Drawing for the job (mm, zero at the part's lowest x, y, z). Coordinates: 2 decimals unless noted, no trailing zeros. Write each loop counter-clockwise with the first axis right and the second up, starting at its lowest first coordinate (ties: lowest second). Pieces come first, ordered by that corner, then holes. Notation, with made-up numbers: (54, 44.5) -> (61, 44.5) arc R27 ccw to (61, 60.5) -> close; hole circle Ø9 at (69, 75). An arc over 180 degrees is marked (long way). Answer as CSV lines item,"result".
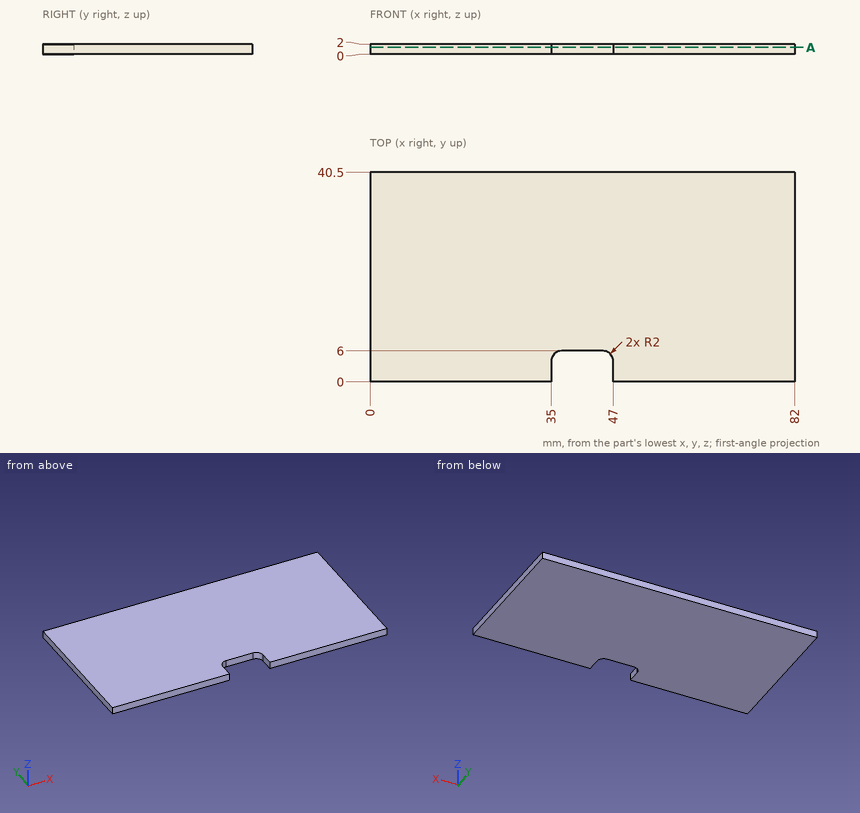
Item 1: Saw through at A-A on z = 1.35. Give the cut face in (x, y), and give its area (3 significant figures).
Answer below:
outline,"(0, 0) -> (35, 0) -> (35, 4) arc R2 cw to (37, 6) -> (45, 6) arc R2 cw to (47, 4) -> (47, 0) -> (82, 0) -> (82, 40.5) -> (0, 40.5) -> close"
area,"3,250 mm2"
Item 2: Flat gauge pins, fed straight in: pin 1 (0.6 mm diameter, centred on x = 42, z = 1, fed in from -Y); pin 2 (1 mm diameter, centred on x = 47, y = 29.5, fed in from -Z). Where does each tip first touch, or does it go through?
Answer below:
pin 1,"stops at y = 6"
pin 2,"stops at z = 0"
Item 3: Wall check: line 1 (X direction, y = 2, z = 0.6); line 2 (Y direction, x = 41, z = 0.35); line 3 (Y direction, x = 35.5, z = 0.5). Give the ranges that are in metal, low to high. Write a range as from..to.
Answer below:
line 1,"x = 0..35, 47..82"
line 2,"y = 6..40.5"
line 3,"y = 5.32..40.5"
